Autodesk Inventor part; units mm, degrees
ref_plane "Plano de trabalho1" through (0, 4, 0) normal (0, 1, 0) x (-1, 0, 0)
ref_plane "YZ Plane" through (0, 0, 0) normal (1, 0, 0) x (0, 1, 0)
ref_plane "XY Plane" through (0, 0, 0) normal (0, 0, 1) x (1, 0, 0)
sketch "Esboço1" plane through (0, 0, 0) normal (0, 0, 1) x (1, 0, 0)
  line L0 (-2.25, 0) -> (-2.25, -10)
  line L1 (-2.25, -10) -> (0, -10)
  line L2 (0, -10) -> (0, 0)
  line L3 (0, 0) -> (0, 4)
  line L4 (-2.25, 0) -> (-4, 0)
  arc A0 (0, 4) -> (-4, 0) centre (0, 0) ccw
  dimension "d1" = 2.25
  dimension "d2" = 10
revolve "Revolução1" add sketch "Esboço1" angle 360 about axis through (0, -10, 0) along (0, 1, 0)
thread "Rosca1"
chamfer "Chanfro1" distance 0.4 angle 45 1 edges at (2.25, -10, 0)
ref_plane "Plano de trabalho1" through (0, 4, 0) normal (0, 1, 0) x (-1, 0, 0)
sketch "Esboço2" plane through (0, 4, 0) normal (0, 1, 0) x (-1, 0, 0)
  line L0 (0.6, -6.0887) -> (-0.6, -6.0887)
  line L1 (-0.6, -6.0887) -> (-0.6, 6.0887)
  line L2 (-0.6, 6.0887) -> (0.6, 6.0887)
  line L3 (0.6, 6.0887) -> (0.6, -6.0887)
  line L4 (0.6, -6.0887) -> (-0.6, 6.0887) construction
  line L5 (-0.6, -6.0887) -> (0.6, 6.0887) construction
  point P0 (0, 0)
  dimension "d10" = 1.2
extrude "Extrusão1" cut sketch "Esboço2" against normal blind 2
properties part number "Parafuso"
Geometry check sheet. Reference: the model listing, model coordinates, mm. A direction names the side the tool comes from. Round coordinates to 2 decimals unless told otherwise and drop trailing zeros. Loops run counter-clockwise (first coordinate to the right, second up) from the corner with the lowest first, then second, coordinate; pieces in that order, holes last. Notation, with made-up numbers: (-35, 13.5) -> (-15, 13.5) arc R19 cw to (-15, 30.5) -> close; hole circle Ø8 at (4, 46). An arc over 180 degrees is marked (long way). Use a Markdown table: item, result.
(1) Scan lines: probe 1 along Y at (x, z) = (-0.5, 0.25); probe 2 along Z at (x, y) = (0, -3.75); probe 3 along Z at (x, y) = (-1.25, -4.25). Record each from-to range of solid material in increasing order.
Calculated:
| item | result |
|---|---|
| probe 1 | -10 to 2 |
| probe 2 | -2.25 to 2.25 |
| probe 3 | -1.87 to 1.87 |
(2) Sectioned sample at A-A (z = 0). Enter the section's corners in (x, y).
Calculated:
| item | result |
|---|---|
| outline | (-4, 0) -> (-2.25, 0) -> (-2.25, -9.6) -> (-1.85, -10) -> (1.85, -10) -> (2.25, -9.6) -> (2.25, 0) -> (4, 0) arc R4 ccw to (0.6, 3.95) -> (0.6, 2) -> (-0.6, 2) -> (-0.6, 3.95) arc R4 ccw to start |
(3) Sectioned sample at C-C (y = -1). Enter the section's corners in (x, z).
Calculated:
| item | result |
|---|---|
| outline | circle Ø4.5 at (0, 0) |
(4) Mould release check, pull along X, two halves, no side actions. Record for faces 3 (the cylindrical face through (0.29, -4.87, -2.23)), 4 (the flat face through (0, -10, 0)), 5 (the flat face through (-0.6, 3, 0)): released by +X, released by -X, zero draft, split by the parting line, or undercut.
Calculated:
| item | result |
|---|---|
| face 3 | split by the parting line |
| face 4 | zero draft |
| face 5 | undercut |
(5) Sectioned sample at D-D (z = 2.5). Enter the section's corners in (x, y) (1 decimal), then the cut area to 3 significant figures.
Calculated:
| item | result |
|---|---|
| outline | (-3.1, 0) -> (3.1, 0) arc R3.1 ccw to (0.6, 3.1) -> (0.6, 2) -> (-0.6, 2) -> (-0.6, 3.1) arc R3.1 ccw to start |
| area | 14.0 mm² |
(6) Sectioned sample at B-B (x = 0). Enter the section's corners in (y, z), then the cut area to 3 significant figures.
Calculated:
| item | result |
|---|---|
| outline | (-10, -1.85) -> (-9.6, -2.25) -> (0, -2.25) -> (0, -4) arc R4 ccw to (2, -3.46) -> (2, 3.46) arc R4 ccw to (0, 4) -> (0, 2.25) -> (-9.6, 2.25) -> (-10, 1.85) -> close |
| area | 60.1 mm² |
(7) Go/stop test with flat-tipped pins: P1, Ø1.5, axis at x = -1.5, y = -1.5, coming from the +Z side; P2, Ø2, axis at y = 2.5, z = 0.5, coming from the -X side; P3, Ø2, axis at y = 1, z = 1, coming from the -X side. Record where each tip stops, or that it passes through.
Calculated:
| item | result |
|---|---|
| P1 | z = 2.12 |
| P2 | x = -3.69 |
| P3 | x = -3.98 |
(8) Set-up check for faces 1 (the flat face through (-2, 0, -2)), 2 (the flat face through (0.6, 3, 0)): record each of +Z, -Z, +X, -X, +Y, -Y from which the full face is reachable in a straight line by a thin tool's end or side.
Calculated:
| item | result |
|---|---|
| face 1 | -Y |
| face 2 | +Z, -Z, +Y |
